```python
from build123d import *

# Parameters (mm, degrees)
SKETCH1_R           = 12.7
BOSS_EXTRUDE1_DEPTH = 177.8
SKETCH4_R           = 10.16
BOSS_EXTRUDE2_DEPTH = 5.08
SKETCH5_R           = 8.128
CUT_EXTRUDE1_DEPTH  = 184.759828036
SKETCH6_R           = 10.287
SKETCH6_R_2         = 8.128
BOSS_EXTRUDE3_DEPTH = 12.7
SKETCH9_W           = 17.78
SKETCH9_H           = 44.45
CUT_EXTRUDE2_DEPTH  = 14.478
FILLET2_R           = 2.54
BOSS_EXTRUDE4_START = -17.78
SKETCH10_R          = 8.128
BOSS_EXTRUDE4_DEPTH = 17.78
SKETCH11_W          = 17.78
SKETCH11_H          = 6.35
CUT_EXTRUDE3_DEPTH  = 9.652
FILLET3_R           = 2.54


with BuildPart() as part:
    # Sketch1 → Boss-Extrude1 (new body)
    with BuildSketch(Plane(origin=(0, 0, 0), x_dir=(1, 0, 0), z_dir=(0, 1, 0))):
        with Locations(Location((0, 0, 0), (0, 0, 270))):
            Circle(SKETCH1_R)
    extrude(amount=BOSS_EXTRUDE1_DEPTH)

    # Sketch4 → Boss-Extrude2 (add)
    with BuildSketch(Plane(origin=(0, 177.8, 0), x_dir=(1, 0, 0), z_dir=(0, 1, 0))):
        with Locations(Location((0, 0, 0), (0, 0, 270))):
            Circle(SKETCH4_R)
    extrude(amount=BOSS_EXTRUDE2_DEPTH)

    # Sketch5 → Cut-Extrude1 (cut, through all)
    with BuildSketch(Plane(origin=(0, 182.88, 0), x_dir=(1, 0, 0), z_dir=(0, 1, 0))):
        with Locations(Location((0, 0, 0), (0, 0, 270))):
            Circle(SKETCH5_R)
    extrude(amount=-CUT_EXTRUDE1_DEPTH, mode=Mode.SUBTRACT)

    # Sketch6 → Boss-Extrude3 (add)
    with BuildSketch(Plane.XZ):
        with Locations(Location((0, 0, 0), (0, 0, 90))):
            Circle(SKETCH6_R)
        with Locations(Location((0, 0, 0), (0, 0, 90))):
            Circle(SKETCH6_R_2, mode=Mode.SUBTRACT)
    extrude(amount=BOSS_EXTRUDE3_DEPTH)


with BuildPart() as body_2:
    # Split1: the piece on the far side of the plane
    add(part.part)
    split(bisect_by=Plane(origin=(0, 2.54, 0), x_dir=(0, 0, -1), z_dir=(0, -1, 0)), keep=Keep.BOTTOM)

    # Sketch9 → Cut-Extrude2 (cut)
    with BuildSketch(Plane(origin=(13.97, 0, 0), x_dir=(0, 0, -1), z_dir=(1, 0, 0))):
        with Locations((0, 27.305)):
            Rectangle(SKETCH9_W, SKETCH9_H)
    extrude(amount=-CUT_EXTRUDE2_DEPTH, mode=Mode.SUBTRACT)

    # Fillet2
    # the kernel refuses this fillet: 2.54 mm, written as the material it takes off along each edge
    with BuildSketch(Plane(origin=(-0.508, 5.08, -8.112109467), x_dir=(-0.988207128280474, 0, 0.15312306036537704), z_dir=(0, 1, 0))) as fillet2_piece_1:
        with BuildLine():
            CenterArc((1.711577927, -2.529447161), FILLET2_R, 95.224634403, 40.891343564)
            Line((-0.119112979, -0.76871697), (-0.155726797, -0.733502366))
            ThreePointArc((-0.155726797, -0.733502366), (-0.109757412, -0.376579834), (-0.050200922, 0.007778651))
            Line((-0.050200922, 0.007778651), (0.004625886, 0.050588943))
            ThreePointArc((0.004625886, 0.050588943), (0.740141806, 0.017030915), (1.475657727, 0.050588943))
            Line((1.475657727, 0.050588943), (1.480283613, 0))
        make_face()
    extrude(amount=44.45, mode=Mode.SUBTRACT)
    with BuildSketch(Plane(origin=(-0.508, 5.08, 8.112109467), x_dir=(-0.9882071282804739, 0, -0.15312306036537726), z_dir=(0, 1, 0))) as fillet2_piece_2:
        with BuildLine():
            CenterArc((1.711577927, 2.529447161), FILLET2_R, 223.884022033, 40.891343564)
            Line((-0.119112979, 0.76871697), (-0.155726797, 0.733502366))
            ThreePointArc((-0.155726797, 0.733502366), (-0.109757412, 0.376579834), (-0.050200922, -0.007778651))
            Line((-0.050200922, -0.007778651), (0.004625886, -0.050588943))
            ThreePointArc((0.004625886, -0.050588943), (0.740141806, -0.017030915), (1.475657727, -0.050588943))
            Line((1.475657727, -0.050588943), (1.480283613, 0))
        make_face()
    extrude(amount=44.45, mode=Mode.SUBTRACT)


with BuildPart() as part_1:
    add(part.part)

    # Split1
    split(bisect_by=Plane(origin=(0, 2.54, 0), x_dir=(0, 0, -1), z_dir=(0, -1, 0)), keep=Keep.TOP)

    add(body_2.part)  # Boss-Extrude4 merges body 2
    # Sketch10 → Boss-Extrude4 (add)
    with BuildSketch(Plane.XZ.offset(12.7).offset(BOSS_EXTRUDE4_START)):
        with Locations(Location((0, 0, 0), (0, 0, 90))):
            Circle(SKETCH10_R)
    extrude(amount=BOSS_EXTRUDE4_DEPTH)

    # Sketch11 → Cut-Extrude3 (cut)
    with BuildSketch(Plane.XY.offset(13.97)):
        with Locations((0, 170.815)):
            Rectangle(SKETCH11_W, SKETCH11_H)
    extrude(amount=-CUT_EXTRUDE3_DEPTH, mode=Mode.SUBTRACT)

    # Fillet3
    # the kernel refuses this fillet: 2.54 mm, written as the material it takes off along each edge
    with BuildSketch(Plane(origin=(-6.88616439, 167.64, 4.318), x_dir=(-1, 0, 0), z_dir=(0, 1, 0))) as fillet3_piece_1:
        with BuildLine():
            CenterArc((3.533151107, -2.028002493), FILLET3_R, 127.019924819, 65.375681648)
            Line((1.052361703, -2.573239995), (1.002745915, -2.584144745))
            ThreePointArc((1.002745915, -2.584144745), (0.589996771, -1.260521604), (-0.043038527, -0.0269875))
            Line((-0.043038527, -0.0269875), (0, 0.0508))
            ThreePointArc((0, 0.0508), (1.001917805, 0.0508), (1.973249301, 0.04056005))
            Line((1.973249301, 0.04056005), (2.00383561, 0))
        make_face()
    extrude(amount=6.35, mode=Mode.SUBTRACT)
    with BuildSketch(Plane(origin=(6.88616439, 167.64, 4.318), x_dir=(0.3785319660304678, 0, -0.9255882187523287), z_dir=(0, 1, 0))) as fillet3_piece_2:
        with BuildLine():
            CenterArc((3.21450585, -2.502579269), FILLET3_R, 99.847172395, 65.375681648)
            Line((0.758515833, -1.854726633), (0.709396033, -1.841769581))
            ThreePointArc((0.709396033, -1.841769581), (0.332238035, -0.946592741), (-0.047019882, -0.019229424))
            Line((-0.047019882, -0.019229424), (0.008687854, 0.050051585))
            ThreePointArc((0.008687854, 0.050051585), (1.390056584, -0.068946339), (2.771425314, 0.050051585))
            Line((2.771425314, 0.050051585), (2.780113168, 0))
        make_face()
    extrude(amount=6.35, mode=Mode.SUBTRACT)


solid = part_1.part
```
Input: part model. Units: mm. Frame: model coordinates. A direction names the side the tool comes from. Coordinates: 2 decimals unless noted, no trailing zeros. Loops run counter-clockwise (first coordinate to the right, second up) from the corner with the lowest first, then second, coordinate; pieces in that order, holes last. Notation, with made-up numbers: (64.25, -1.75) -> (101.25, -1.75) arc R14 cw to (101.25, 25.25) -> close; hole circle Ø1 at (78.25, 27). An arc over 180 degrees is marked (long way). Use a Markdown table: item, result.
1) Contact query for flat-ended pins moving along their axis: pin 1 (3 mm diameter, centred on x = 5.5, z = 2.5, fed in from +Y); pin 2 (1.5 mm diameter, centred on y = 23, z = -8.5, fed in from +X); pin 3 (8 mm diameter, centred on y = 86.5, z = -5, fed in from +X). Output: stop coordinate, or through.
Results found:
| item | result |
|---|---|
| pin 1 | stops at y = 5.08 |
| pin 2 | stops at x = 9.07 |
| pin 3 | stops at x = 12.66 |
2) Cut plane A-A (z = 0). Return the cut outline in (x, y), then the cut area to 3 significant figures.
Results found:
| item | result |
|---|---|
| outline | (-12.7, 0) -> (-10.29, 0) -> (-10.29, -12.7) -> (10.29, -12.7) -> (10.29, 0) -> (12.7, 0) -> (12.7, 5.08) -> (-8.13, 5.08) -> (-8.13, 182.88) -> (-10.16, 182.88) -> (-10.16, 177.8) -> (-12.7, 177.8) -> close; (8.13, 49.53) -> (12.7, 49.53) -> (12.7, 177.8) -> (10.16, 177.8) -> (10.16, 182.88) -> (8.13, 182.88) -> close |
| area | 1,790 mm2 |
3) Pull-direction query (Z, two-part tool) for faces 6 (the cylindrical face through (-8.06, 95.22, -1.06)), 7 (the flat face through (0, 167.64, 9)), 8 (the cylindrical face through (-10.2, -6.26, -1.34)); classes: released by +Z, released by -Z, zero draft, split by the parting line, or undercut.
Results found:
| item | result |
|---|---|
| face 6 | undercut |
| face 7 | zero draft |
| face 8 | split by the parting line |
4) Material intervals for line 1 along Y through (x, z) = (7.75, -5.75); line 2 along Y through (x, z) = (7.25, -8.25); line 3 along X through (y, z) = (144, 0), sorted ascending. Write a range as from..to.
Results found:
| item | result |
|---|---|
| line 1 | y = -12.7..5.08, 49.53..182.88 |
| line 2 | y = 0..5.08, 49.53..177.8 |
| line 3 | x = -12.7..-8.13, 8.13..12.7 |
5) Cut plane B-B (x = 4). Return the cut outline in (y, z), then the cut area to 3 significant figures.
Results found:
| item | result |
|---|---|
| outline | (-12.7, -9.48) -> (0, -9.48) -> (0, -12.05) -> (177.8, -12.05) -> (177.8, -9.34) -> (182.88, -9.34) -> (182.88, -7.08) -> (49.53, -7.08) -> (49.53, -8.89) -> (5.08, -8.89) -> (5.08, 8.89) -> (49.53, 8.89) -> (49.53, 7.08) -> (167.64, 7.08) -> (167.64, 12.05) -> (0, 12.05) -> (0, 9.48) -> (-12.7, 9.48) -> close; (173.99, 7.08) -> (182.88, 7.08) -> (182.88, 9.34) -> (177.8, 9.34) -> (177.8, 12.05) -> (173.99, 12.05) -> close |
| area | 1,910 mm2 |
6) Access query for faces 1 (the flat face through (2, 5.08, 0)), 2 (the cylindrical face through (-12.4, 87.66, -2.75)), 3 (the flat face through (-9.35, 0, 4.64)), 4 (the flat face through (8.89, 171, 7)), 5 (the cylindrical face through (10.074, 180.304, -1.323)). Directions: +Z, -Z, +X, -X, +Y, -Y. A direction counts if a zero-diameter tool reaches every point of the face in a straight line with its end or side. Return the directions, or none.
Results found:
| item | result |
|---|---|
| face 1 | +X |
| face 2 | +Y, -Y |
| face 3 | -Y |
| face 4 | +Z |
| face 5 | +Y |
7) Cut plane D-D (y = 39.5). Return the cut outline in (x, z).
Results found:
| item | result |
|---|---|
| outline | (-1.97, -7.89) arc R8.13 cw to (-1.97, 7.89) arc R2.54 ccw to (-0.51, 8.89) -> (9.07, 8.89) arc R12.7 ccw (long way) to (9.07, -8.89) -> (-0.51, -8.89) arc R2.54 ccw to start |
8) Cut plane C-C (y = 91). Return the cut outline in (x, z), then the cut area to 3 significant figures.
Results found:
| item | result |
|---|---|
| outline | circle Ø25.4 at (0, 0); hole circle Ø16.26 at (0, 0) |
| area | 299 mm2 |
